Autodesk Inventor part; units mm, degrees
ref_plane "YZ Plane" through (0, 0, 0) normal (1, 0, 0) x (0, 1, 0)
ref_plane "XZ Plane" through (0, 0, 0) normal (0, 1, 0) x (-1, 0, 0)
ref_plane "XY Plane" through (0, 0, 0) normal (0, 0, 1) x (1, 0, 0)
sketch "Skizze1" plane through (0, 0, 0) normal (0, 0, 1) x (1, 0, 0)
  line L0 (-25, 5) -> (25, 5)
  line L1 (25, 5) -> (25, -5)
  line L2 (25, -5) -> (-25, -5)
  line L3 (-25, -5) -> (-25, 5)
  line L4 (-25, 5) -> (25, -5) construction
  line L5 (25, 5) -> (-25, -5) construction
  point P0 (0, 0)
  dimension "d0" = 50
  dimension "d1" = 10
extrude "Extrusion1" add sketch "Skizze1" along normal mid plane 500
sketch "Skizze4" plane through (-25, -5, 250) normal (0, -1, 0) x (1, 0, 0)
  line L0 (50, -500) -> (50, 0)
  line L1 (0, 0) -> (50, 0)
  line L2 (0, 0) -> (0, -500)
  line L3 (50, -500) -> (0, -500)
  point P0 (25, -250)
  point P1 (30, -465)
  dimension "d13" = 30
  dimension "d14" = 35
hole "Bohrung2" [suppressed]
sketch "Skizze5" plane through (-25, -5, 250) normal (0, -1, 0) x (1, 0, 0)
  line L0 (50, -500) -> (50, 0)
  line L1 (0, 0) -> (50, 0)
  line L2 (0, 0) -> (0, -500)
  line L3 (50, -500) -> (0, -500)
  point P0 (25, -250)
  point P1 (6, -250)
  point P2 (0, -250)
  dimension "d22" = 6
hole "Bohrung3" at (-19, -5, 0) direction (0, 1, 0) diameter 5.5 depth 32.3 tip angle 118 counterbore diameter 10 counterbore depth 5
pattern_linear "Rechteckige Anordnung1" count 3 spacing 110 along (0, 0, -1) count 3 spacing 110 along (0, 0, 1) of "Bohrung3"
sketch "Skizze6" plane through (25, 5, 250) normal (1, 0, 0) x (0, 0, -1)
  line L0 (500, 0) -> (0, 0)
  line L1 (0, -10) -> (0, 0)
  line L2 (500, -10) -> (0, -10)
  line L3 (500, 0) -> (500, -10)
  point P0 (250, -5)
  point P1 (250, -4)
  dimension "d60" = 6
hole "Bohrung4" at (25, 1, 0) direction (-1, 0, 0) diameter 4.134 depth 14.2 tip angle 118
pattern_linear "Rechteckige Anordnung2" count 3 spacing 110 along (0, 0, 1) count 3 spacing 110 along (0, 0, -1) of "Bohrung4"
sketch "Skizze7" plane through (0, 0, 250) normal (0, 0, 1) x (1, 0, 0)
  line L0 (-21.75, 5) -> (-21.75, 0)
  line L1 (-25, 5) -> (-25, -5)
  line L2 (25, 5) -> (-25, 5)
  point P0 (0, 0)
  point P1 (-19, 1)
  dimension "d49" = 6
  dimension "d61" = 4
hole "Bohrung5" at (-19, 1, 250) direction (0, 0, -1) diameter 4.134 depth 14.2 tip angle 118
chamfer "Fasen1" distance 0.5 angle 45 1 edges at (-19, 3.067, 250)
properties part number "Platte-2"
Build history of the part. All positions in model axes, mm. A direction names the side the tool comes from. Round coordinates to 2 decimals unless told otherwise and drop trailing zeros.
Item 1: Pin check, flat tips, straight feed: P1, Ø5, axis at y = 1, z = -220, coming from the +X side; P2, Ø5, axis at x = -20, z = 111, coming from the -Y side; P3, Ø3.5, axis at y = 1, z = -110, coming from the +X side. Stop position of each tip, or through.
Item 2: Drill centre lines: line 1 along Z through (x, y) = (-19, 3.7); line 2 along Z through (x, y) = (-19, -3.85); line 3 along X through (y, z) = (4, 110). Where is each one in solid material? Low to high.
Item 3: Which spindle directions (+Z, -Z, +X, -X, +Y, -Y) get a long thin tool onto all of the face, cutting with end or side? Do faces 5 (the face through (-16.8, 0, -2.2)), 6 (the face through (0, 5, -4)). Say none if no direction does.
Item 4: Two-plate mould, pull along Z, no slides. Class faces 1 (the face through (-17.085, -2.465, 105.381)), 2 (the face through (25, 0, -4)), 3 (the face through (-14.12, -2.46, 1.08)), 4 (the face through (0, 0, -250)): released by +Z, released by -Z, zero draft, split by the parting line, or undercut.
Worked answers:
1. P1: stops at x = 25
1. P2: stops at y = 0
1. P3: stops at x = 10.61
2. line 1: z = -250 to -222.75, -217.25 to -112.75, -107.25 to -2.75, 2.75 to 107.25, 112.75 to 217.25, 222.75 to 250
2. line 2: z = -250 to -225, -215 to -115, -105 to -5, 5 to 105, 115 to 215, 225 to 250
2. line 3: x = -25 to -21.75, -16.25 to 25
3. face 5: -Y
3. face 6: +Z, -Z, +X, -X, +Y
4. face 1: undercut
4. face 2: zero draft
4. face 3: undercut
4. face 4: released by -Z
